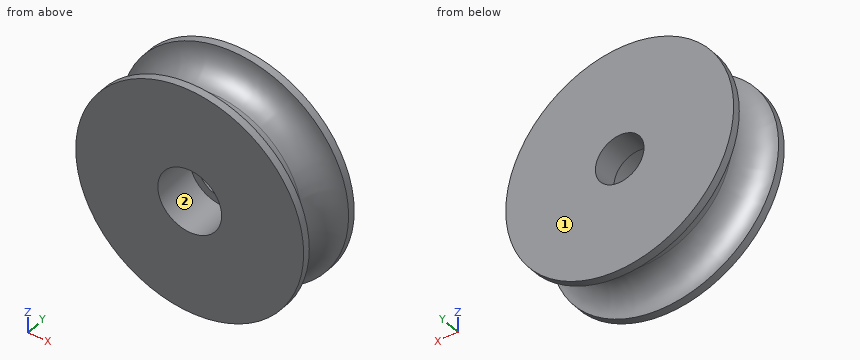
```python
from build123d import *

# Parameters (mm, degrees)
F0_R       = 75
F1_DEPTH   = 22.5
F2_R       = 17.5
F5_R       = 21
F6_DEPTH   = 28.5
F7_R       = 16
F1_FACE1_R = 75
F8_DEPTH   = 45.001


with BuildPart() as f1:
    # F0 (on Front) → F1 (new body, symmetric)
    with BuildSketch(Plane.XZ):
        Circle(F0_R)
    extrude(amount=F1_DEPTH, both=True)

    # F2 (on Top) → F4 (revolve, cut)
    with BuildSketch(Plane.XY):
        with Locations((-75, 0)):
            Circle(F2_R)
    revolve(axis=Axis((0, 4.404310137, 0), (0, -1, 0)), mode=Mode.SUBTRACT)

    # F5 (on face) → F6 (cut)
    with BuildSketch(Plane.XZ.offset(22.5)):
        Circle(F5_R)
    extrude(amount=-F6_DEPTH, mode=Mode.SUBTRACT)

    # F7 (on face) + F1_face1 (on face) → F8 (cut, through all)
    with BuildSketch(Plane.XZ.offset(22.5)):
        Circle(F7_R)
    with BuildSketch(Plane(origin=(0, 22.5, 0), x_dir=(1, 0, 0), z_dir=(0, 1, 0))):
        Circle(F1_FACE1_R)
    extrude(amount=-F8_DEPTH, dir=(0, -1, 0), mode=Mode.SUBTRACT)


solid = f1.part
```
Here's how the part is built. I have some questions about the finished solid (model axes, mm). Face numbers are marked on the shaded views. Round coordinates to 2 decimals unless told otherwise and drop trailing zeros. Order: outer loops, then holes, each group sorted by start corner. A loop starts at its lowest first (then second) coordinate and runs counter-clockwise, first axis right, second up. Notation, with made-up numbers: M 2,50 L 24,50 A27 cw 24,87 Z; hole C 61,-38 d9. An arc over 180 degrees is marked long. Answer in a Markdown table with one row per item.
Item 1: Imagine slicing it at D-D, the plane y = 13. Write out the boundary of the cut face in (x, z), and give its area (3 significant figures).
A:
| item | result |
|---|---|
| outline | C 0,0 d126.57; hole C 0,0 d32 |
| area | 11,800 mm2 |
Item 2: Imagine slicing it at C-C, the plane y = -14. Write out the boundary of the cut face in (x, z).
A:
| item | result |
|---|---|
| outline | C 0,0 d129; hole C 0,0 d42 |
Item 3: Imagine slicing it at A-A, the plane z = 0. Write out the boundary of the cut face in (x, y), and give its area (3 significant figures).
A:
| item | result |
|---|---|
| outline | M -75,-22.5 L -21,-22.5 L -21,6 L -16,6 L -16,22.5 L -75,22.5 L -75,17.5 A17.5 cw -75,-17.5 Z; M 16,6 L 21,6 L 21,-22.5 L 75,-22.5 L 75,-17.5 A17.5 cw 75,17.5 L 75,22.5 L 16,22.5 Z |
| area | 4,060 mm2 |
Item 4: Thinking about a two-plate mould opening in Z: for the marked faces 1 and 2, which applies, +Z half, -Z half, draft (parallel to the pull), parting line (faces both ways), or undercut?
A:
| item | result |
|---|---|
| face 1 | draft |
| face 2 | undercut |
Item 5: If I drill on L1, parallel to Z at x = 0, y = 19; L2, parallel to Y at x = 69, z = 28; L3, parallel to Y at x = -7.5, z = -15.5, over which ranges is the centre line in solid material (lowest first)? Write a range as from..to.
A:
| item | result |
|---|---|
| L1 | z = -75..-16, 16..75 |
| L2 | y = -22.5..-17.49, 17.49..22.5 |
| L3 | y = 6..22.5 |
Item 6: I'm going to push flat-ended pins straight in: pin 1 (2 mm diameter, centred on y = -3.5, z = 18, fed in from +X); pin 2 (12 mm diameter, centred on x = -6.5, y = 1.5, fed in from -Z); pin 3 (4 mm diameter, centred on x = -15.5, y = -1.5, fed in from -Z). Where does each tip first touch, or does it pass through?
A:
| item | result |
|---|---|
| pin 1 | stops at x = 55.38 |
| pin 2 | stops at z = -58.89 |
| pin 3 | stops at z = -56.01 |
Item 7: Imagine slicing it at B-B, the plane x = 0. Write out the boundary of the cut face in (y, z), and give its area (3 significant figures).
A:
| item | result |
|---|---|
| outline | M -22.5,-75 L -17.5,-75 A17.5 cw 17.5,-75 L 22.5,-75 L 22.5,-16 L 6,-16 L 6,-21 L -22.5,-21 Z; M -22.5,21 L 6,21 L 6,16 L 22.5,16 L 22.5,75 L 17.5,75 A17.5 cw -17.5,75 L -22.5,75 Z |
| area | 4,060 mm2 |
